Can you work these out from the model? Positions are in its coordinate system, mm. A direction names the side the tool comes from. Give positions to 0.01 mm unless a question says otherwise; leave off trailing zeros. Return JSON: item names as keys, results as strings. Group by question number.
Q1. Thinking about a two-plate mould opening in Z: for faces 4 (the cylindrical face through (43.93, -0.9, 2.86)), 5 (the flat face through (39, 2.5, -2.5)), 6 (the cylindrical face through (35.81, 1.03, 8.85)), which applies, pulls with the +Z half, pulls with the -Z half, needs draft (parallel to the pull), parting line crosses it, or undercut?
Q2. I need wall thicknesses on line 1 along Y through (x, z) = (35.65, 0); line 2 along X through (y, z) = (5.5, 3); line 3 along Z through (x, y) = (20, -0.25). Which ranges of each line are inside material? Lowest first, please. Write a range as [from, to].
Q3. Will these pins go through, and if not, where does the flat tip stop? pin 1 (8 mm diameter, centred on x = 9.5, z = -9, fed in from -Y); pin 2 (4.5 mm diameter, centred on y = 0, z = 7.5, fed in from +X); pin 3 (5 mm diameter, centred on y = -6, z = -2.5, fed in from +X); pin 4 (6 mm diameter, centred on x = 29.5, z = 5, fed in from +Y).
Q4. Which directions (+Z, -Z, +X, -X, +Y, -Y) give clear straight access to the entire face, cutting with the end or side of a thin tool? Please do faces 1 (the flat face through (36.6, 1.4, -6.1)), 2 (the flat face through (35, 0, 5)), 3 (the flat face through (49, 0, 0)).
Q5. Suppose I cut it at A-A, the plane y = 0. Count the separate pieces of the cut face and the enclosed holes in it, and give its area (3 significant figures).
```python
from build123d import *

# Parameters (mm, degrees)
CBORE_FOR_M3_HEX_SOCKET_THIN_HEAD_CA_2_COUNT = 2
CBORE_FOR_M3_HEX_SOCKET_THIN_HEAD_CA_2_PITCH = 10.606601718
CBORE_FOR_M3_HEX_SOCKET_THIN_HEAD_CA_3_COUNT = 2
CBORE_FOR_M3_HEX_SOCKET_THIN_HEAD_CA_3_PITCH = 15
CBORE_FOR_M3_HEX_SOCKET_THIN_HEAD_CA_4_COUNT = 2
CBORE_FOR_M3_HEX_SOCKET_THIN_HEAD_CA_4_PITCH = 10.606601718


with BuildPart() as part:
    # Sketch1 → Revolve1 (revolve)
    with BuildSketch(Plane.XY, mode=Mode.PRIVATE) as revolve1_sk:
        Polygon((49, 0), (49, 3), (39, 3), (39, 12), (35, 12), (35, 4.5), (0, 4.5), (0, 0), align=None)
    revolve(revolve1_sk.sketch.rotate(Axis((0, 0, 0), (1, 0, 0)), 90), axis=Axis((0, 0, 0), (1, 0, 0)))

    # Sketch3 → CBORE for M3 Hex Socket Thin Head Cap Screw1 (revolve, cut)
    with BuildSketch(Plane(origin=(39, 0, 7.5), x_dir=(0, 0, -1), z_dir=(0, 1, 0))):
        Polygon((0, 0), (0, 39), (1.7, 39), (1.7, 2.4), (3.25, 2.4), (3.25, 0.025), (3.275, 0), align=None)
    cbore_for_m3_hex_socket_thin_head_cap_sc = revolve(axis=Axis((45.35, 0, 7.5), (-1, 0, 0)), mode=Mode.SUBTRACT)

    # CBORE for M3 Hex Socket Thin Head Ca 2: CBORE for M3 Hex Socket Thin Head Cap Screw1 ×2
    with Locations(*[Vector(0, 0.7071067811865674, -0.7071067811865277) * (i * CBORE_FOR_M3_HEX_SOCKET_THIN_HEAD_CA_2_PITCH) for i in range(1, CBORE_FOR_M3_HEX_SOCKET_THIN_HEAD_CA_2_COUNT)]):
        add(cbore_for_m3_hex_socket_thin_head_cap_sc, mode=Mode.SUBTRACT)

    # CBORE for M3 Hex Socket Thin Head Ca 3: CBORE for M3 Hex Socket Thin Head Cap Screw1 ×2
    with Locations(*[(0, 0, -i * CBORE_FOR_M3_HEX_SOCKET_THIN_HEAD_CA_3_PITCH) for i in range(1, CBORE_FOR_M3_HEX_SOCKET_THIN_HEAD_CA_3_COUNT)]):
        add(cbore_for_m3_hex_socket_thin_head_cap_sc, mode=Mode.SUBTRACT)

    # CBORE for M3 Hex Socket Thin Head Ca 4: CBORE for M3 Hex Socket Thin Head Cap Screw1 ×2
    with Locations(*[Vector(0, -0.7071067811865276, -0.7071067811865674) * (i * CBORE_FOR_M3_HEX_SOCKET_THIN_HEAD_CA_4_PITCH) for i in range(1, CBORE_FOR_M3_HEX_SOCKET_THIN_HEAD_CA_4_COUNT)]):
        add(cbore_for_m3_hex_socket_thin_head_cap_sc, mode=Mode.SUBTRACT)


solid = part.part
```
Ans:
{
 "1": {"face 4": "parting line crosses it", "face 5": "needs draft", "face 6": "undercut"},
 "2": {"line 1": "y = [-12, -9.2], [-5.8, 5.8], [9.2, 12]", "line 2": "x = [35, 39]", "line 3": "z = [-4.49, 4.49]"},
 "3": {"pin 1": "passes through", "pin 2": "stops at x = 36.6", "pin 3": "stops at x = 39", "pin 4": "stops at y = 4.03"},
 "4": {"face 1": "+X", "face 2": "-X", "face 3": "+Z, -Z, +X, +Y, -Y"},
 "5": {"separate pieces": "3", "enclosed holes": "0", "area": "429 mm^2"}
}
